Design review of the part shown in the three views and the two pictorial views. Dimensions are in mm from the part's minimum x, y and z. A direction names the side the tool comes from. Give positions to 0.01 mm unless a question says otherwise; leave off trailing zeros. Loops run counter-clockwise (first coordinate to the right, second up) from the corner with the lowest first, then second, coordinate; pieces in that order, holes last. Notation, with made-up numbers: (-30.75, 61) - (-1.75, 61) arc R24 cw to (-1.75, 76) - close; hole circle Ø5 at (-11, 36.5). An arc over 180 degrees is marked (long way). Put each result on its own line as item: value. Start each with the question number.
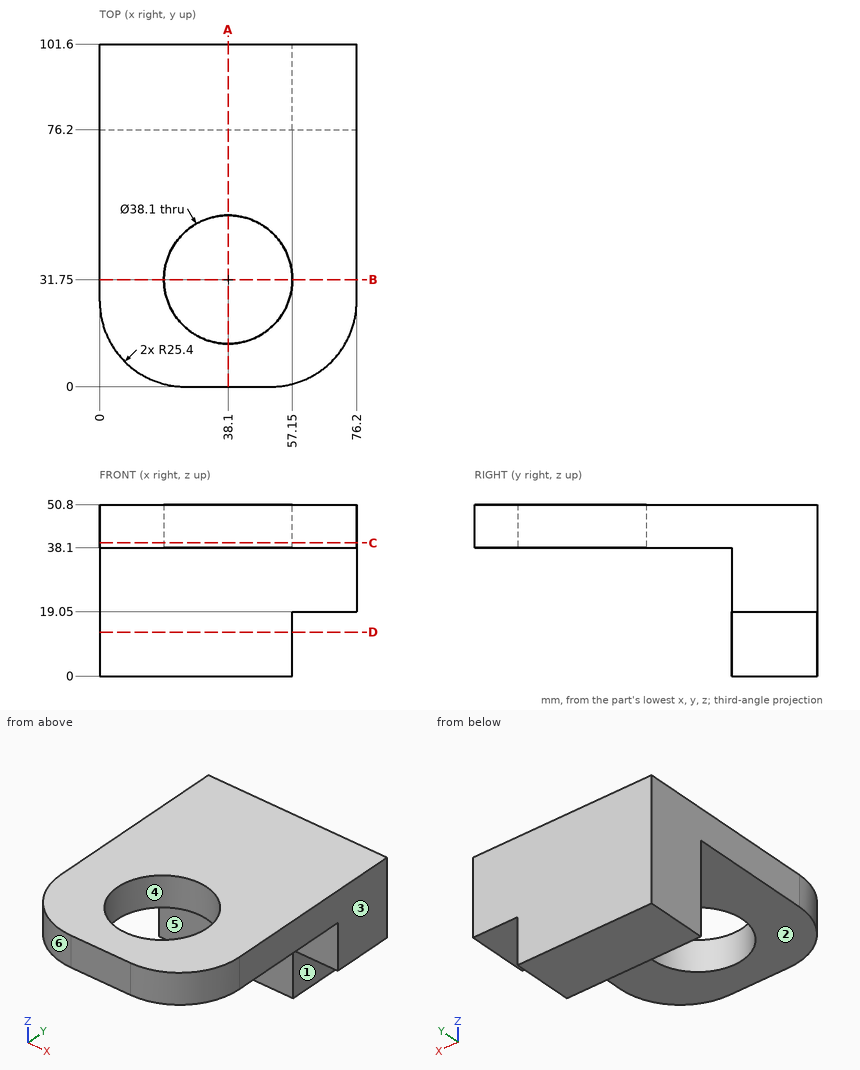
1) Take a section at B-B on y = 31.75. State the section outline as (x, z) points.
2) Machinability: for the marked faces 1, 2 and 3, which of the approach directions +Z, -Z, +X, -X, +Y, -Y give a long, thin tool a straight path to every point of the face, cutting with its end or side? Answer none if there is none.
3) Take a section at D-D on z = 13. State the section outline as (x, y) points.
4) Take a section at C-C on z = 39.5. State the section outline as (x, y) points, and give its area (3 significant figures).
5) Mouldability with a two-part tool opening along X and no side actions: class the marked faces 4, 5 and 6 as released by +X, released by -X, zero draft, split by the parting line, or undercut.
6) Take a section at A-A on x = 38.1. State the section outline as (y, z) points.
7) Wall thickness on probe 1 along Y at (x, z) = (38, 41); probe 2 along X at (y, z) = (31, 44); probe 3 along Y at (x, z) = (59, 31.5): over which ranges is each line inside the solid? List them lowest first.
8) Insertion check: P1, Ø1, axis at x = 63.5, z = 35, coming from the -Y side; P2, Ø21, axis at y = 91.5, z = 5.5, coming from the +X side; P3, Ø5, axis at x = 46.5, y = 47.5, coming from the +Z side. Each pin has a flat end and moves straight along its axis. Give the tip position at first contact, or say it passes through.
Answers follow:
1. outline: (0, 38.1) - (19.05, 38.1) - (19.05, 50.8) - (0, 50.8) - close; (57.15, 38.1) - (76.2, 38.1) - (76.2, 50.8) - (57.15, 50.8) - close
2. face 1: -Z, +X, +Y, -Y
2. face 2: -Z, +X, -X, -Y
2. face 3: +Z, -Z, +X, +Y, -Y
3. outline: (0, 76.2) - (57.15, 76.2) - (57.15, 101.6) - (0, 101.6) - close
4. outline: (0, 25.4) arc R25.4 ccw to (25.4, 0) - (50.8, 0) arc R25.4 ccw to (76.2, 25.4) - (76.2, 101.6) - (0, 101.6) - close; hole circle Ø38.1 at (38.1, 31.75)
4. area: 6,320 mm2
5. face 4: undercut
5. face 5: zero draft
5. face 6: released by -X
6. outline: (0, 38.1) - (12.7, 38.1) - (12.7, 50.8) - (0, 50.8) - close; (50.8, 38.1) - (76.2, 38.1) - (76.2, 0) - (101.6, 0) - (101.6, 50.8) - (50.8, 50.8) - close
7. probe 1: 0 to 12.7, 50.8 to 101.6
7. probe 2: 0 to 19.06, 57.14 to 76.2
7. probe 3: 76.2 to 101.6
8. P1: y = 76.2
8. P2: x = 57.15
8. P3: z = 50.8
